The drawing under review shows one solid part. Ordinate dimensions are in mm from its lowest x, y, z. A direction names the side the tool comes from. Coordinates: 2 decimals unless noted, no trailing zeros. Loops run counter-clockwise (first coordinate to the right, second up) from the corner with the lowest first, then second, coordinate; pieces in that order, holes last. Notation, with made-up numbers: M -4,30.5 L 21,30.5 A19 cw 21,61.5 Z; hole C 80,68 d3. An arc over 180 degrees is marked long. Put each result on its own line as item: value.
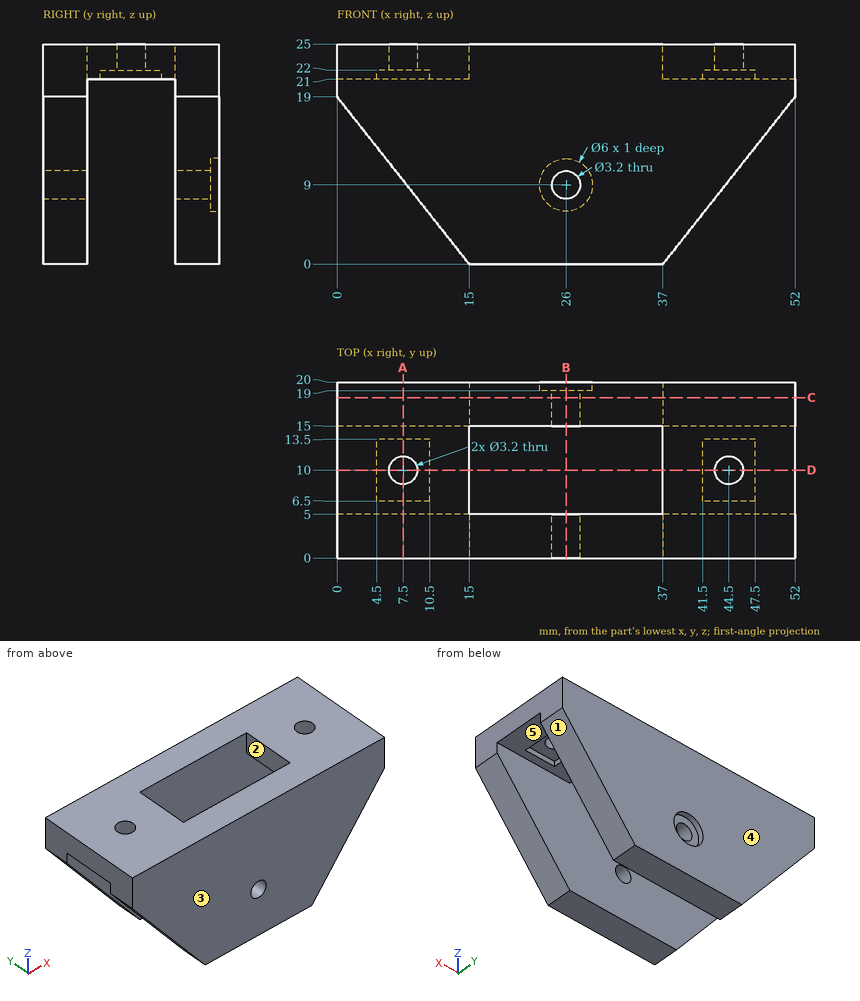
(1) Add section A-A (x = 7.5). Write out the cut boundary in (y, z).
Determined:
outline: M 0,9.5 L 5,9.5 L 5,21 L 6.5,21 L 6.5,22 L 8.4,22 L 8.4,25 L 0,25 Z; M 11.6,22 L 13.5,22 L 13.5,21 L 15,21 L 15,9.5 L 20,9.5 L 20,25 L 11.6,25 Z
(2) Tool access review of the marked faces 4 and 5: name each direction out of +Z, -Z, +X, -X, +Y, -Y from which nothing blocks a thin tool from reaching the whole face with its end or side.
Determined:
face 4: +Z, -Z, +X, -X, +Y
face 5: -Z, +X, -X
(3) Add section D-D (y = 10). Write out the cut boundary in (x, z).
Determined:
outline: M 0,21 L 4.5,21 L 4.5,22 L 5.9,22 L 5.9,25 L 0,25 Z; M 9.1,22 L 10.5,22 L 10.5,21 L 15,21 L 15,25 L 9.1,25 Z; M 37,21 L 41.5,21 L 41.5,22 L 42.9,22 L 42.9,25 L 37,25 Z; M 46.1,22 L 47.5,22 L 47.5,21 L 52,21 L 52,25 L 46.1,25 Z
(4) Add section C-C (y = 18.25). Write out the cut boundary in (x, z).
Determined:
outline: M 0,19 L 15,0 L 37,0 L 52,19 L 52,25 L 0,25 Z; hole C 26,9 d3.2
(5) Add section B-B (x = 26). Write out the cut boundary in (y, z), plus the area to 3 significant figures.
Determined:
outline: M 0,0 L 5,0 L 5,7.4 L 0,7.4 Z; M 0,10.6 L 5,10.6 L 5,25 L 0,25 Z; M 15,0 L 20,0 L 20,6 L 19,6 L 19,7.4 L 15,7.4 Z; M 15,10.6 L 19,10.6 L 19,12 L 20,12 L 20,25 L 15,25 Z
area: 215 mm^2
(6) For pin 1 (10 mm diameter, centred on y = 4, z = 3.5, fed in from +X); pin 2 (3 mm diameter, centred on x = 7.5, y = 10, fed in from +Z); pin 3 (8 mm diameter, centred on y = 15, z = 14, fed in from +X); pin 4 (5 mm diameter, centred on x = 45.5, y = 11.5, fed in from -Z), all flat-tipped, find the tip position at first contact; note any pin that passes through.
Determined:
pin 1: stops at x = 43.71
pin 2: passes through
pin 3: stops at x = 51.21
pin 4: stops at z = 21
(7) Wall thickness on line 1 along X through (y, z) = (10, 23.1); line 2 along Y through (x, z) = (38, 17.75); line 3 along Z through (x, y) = (26, 19.6): over which ranges is each line inside the solid? List them lowest first. Write a range as [from, to].
Determined:
line 1: x = [0, 5.9], [9.1, 15], [37, 42.9], [46.1, 52]
line 2: y = [0, 5], [15, 20]
line 3: z = [0, 6], [12, 25]
(8) Draft analysis for pull direction X (two halves, no side actions). For the marked faces 1, 2 and 3, state which applies: +X half, -X half, draft (parallel to the pull), parting line (faces both ways), or undercut.
Determined:
face 1: +X half
face 2: undercut
face 3: draft
